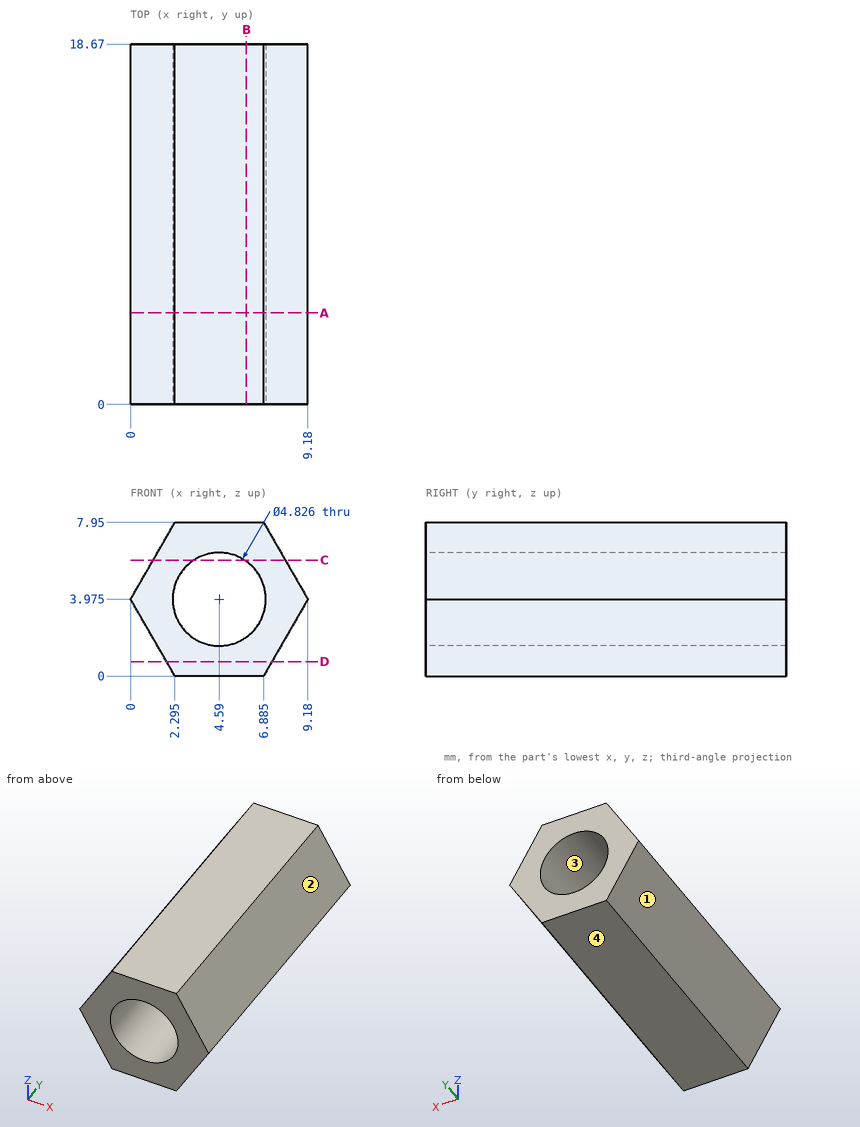
Study the drawing (mm; zero at the part's minimum x, y, z) and answer. Round coordinates to 2 decimals unless told otherwise and drop trailing zeros. Order: outer loops, then holes, each group sorted by start corner. A loop starts at its lowest first (then second) coordinate and runs counter-clockwise, first axis right, second up. Notation, with made-up numbers: M 22.25,18 L 56.25,18 A30 cw 56.25,44 Z; hole C 82.5,-31 d3. An arc over 180 degrees is marked long. One line per item, written item: value.
Q1. Find section C-C on z = 6. Write down the section's boundary in (x, y).
Derived:
outline: M 1.17,0 L 3.28,0 L 3.28,18.67 L 1.17,18.67 Z; M 5.9,0 L 8.01,0 L 8.01,18.67 L 5.9,18.67 Z
Q2. Find section A-A on y = 4.75. Write down the section's boundary in (x, z) (3 decimals).
Derived:
outline: M 0,3.975 L 2.295,0 L 6.885,0 L 9.18,3.975 L 6.885,7.95 L 2.295,7.95 Z; hole C 4.59,3.975 d4.826
Q3. Find section D-D on z = 0.75. Write down the section's boundary in (x, y).
Derived:
outline: M 1.86,0 L 7.32,0 L 7.32,18.67 L 1.86,18.67 Z
Q4. Flat-ended cylindrical pins translate along their axes: pin 1 (3 mm diameter, centred on x = 3.5, z = 6, fed in from -Y); pin 2 (4 mm diameter, centred on x = 4.59, z = 3.98, fed in from +Y). Find the tip coordinate at first contact, or state that the pin passes through.
Derived:
pin 1: y = 0
pin 2: through
Q5. Determine the mould class of the marked faces 1, 2, 3 and 4 for opening direction X: released by +X, released by -X, zero draft, split by the parting line, or undercut.
Derived:
face 1: released by -X
face 2: released by +X
face 3: undercut
face 4: zero draft
Q6. Find section B-B on x = 6. Write down the section's boundary in (y, z).
Derived:
outline: M 0,0 L 18.67,0 L 18.67,2.02 L 0,2.02 Z; M 0,5.93 L 18.67,5.93 L 18.67,7.95 L 0,7.95 Z
Q7. Straight lines are drawn through the part: line 1 (Z direction, x = 5.5, y = 5.75); line 2 (X direction, y = 3.5, z = 6); line 3 (Z direction, x = 6, y = 1.5). For each, find the intervals that lie inside material, in ascending order.
Derived:
line 1: 0 to 1.74, 6.21 to 7.95
line 2: 1.17 to 3.28, 5.9 to 8.01
line 3: 0 to 2.02, 5.93 to 7.95
